Geometry check sheet. Reference: the model listing, model coordinates, mm. A direction names the side the tool comes from. Give positions to 0.01 mm unless a question says otherwise; leave off trailing zeros. Loops run counter-clockwise (first coordinate to the right, second up) from the corner with the lowest first, then second, coordinate; pieces in that order, holes last. Notation, with made-up numbers: (29, 85.5) - (76, 85.5) arc R20 cw to (76, 91.5) - close; hole circle Ø2 at (87.25, 71). An arc over 180 degrees is marked (long way). One line per question, with ' | ' between items. Start each with the question number.
Autodesk Inventor part; units mm, degrees
ref_plane "YZ Plane" through (0, 0, 0) normal (1, 0, 0) x (0, 1, 0)
ref_plane "XZ Plane" through (0, 0, 0) normal (0, 1, 0) x (-1, 0, 0)
ref_plane "XY Plane" through (0, 0, 0) normal (0, 0, 1) x (1, 0, 0)
sketch "Sketch1" plane through (0, 0, 0) normal (0, 0, 1) x (1, 0, 0)
  line L0 (0, 0) -> (50.8, 0)
  line L1 (50.8, 0) -> (50.8, 25.4)
  line L2 (50.8, 25.4) -> (0, 25.4)
  line L3 (0, 25.4) -> (0, 0)
  line L4 (1.905, 23.495) -> (48.895, 23.495)
  line L5 (48.895, 23.495) -> (48.895, 1.905)
  line L6 (48.895, 1.905) -> (1.905, 1.905)
  line L7 (1.905, 1.905) -> (1.905, 23.495)
  dimension "d0" = 50.8
  dimension "d1" = 25.4
  dimension "d2" = 1.905
extrude "Extrusion1" add sketch "Sketch1" along normal blind 330.2
sketch "Sketch2" plane through (0, 25.4, 0) normal (0, 1, 0) x (1, 0, 0)
  line L0 (1.905, -330.2) -> (48.895, -330.2) construction
  line L1 (25.4, -330.2) -> (25.4, -304.8) construction
  line L2 (25.4, -304.8) -> (25.4, -228.6) construction
  line L3 (50.8, 0) -> (0, 0) construction
  line L4 (25.4, 0) -> (25.4, -25.4) construction
  circle A0 centre (25.4, -304.8) radius 14.2748
  circle A1 centre (25.4, -25.4) radius 14.2875
  line L5 (25.4, -228.6) -> (12.7, -228.6) construction
  line L6 (12.7, -228.6) -> (25.4, -228.6) construction
  line L7 (25.4, -228.6) -> (38.1, -228.6) construction
  circle A2 centre (12.7, -228.6) radius 2.5797
  circle A3 centre (38.1, -228.6) radius 2.5797
  dimension "d5" = 25.4
  dimension "d6" = 76.2
  dimension "d7" = 25.4
  dimension "d8" = 28.5496
  dimension "d9" = 28.575
  dimension "d10" = 12.7
  dimension "d11" = 12.7
  dimension "d12" = 5.1594
  dimension "d13" = 5.1594
extrude "Extrusion2" cut sketch "Sketch2" against normal blind 355.6
properties part number "arm"
(1) Section check C-C, the plane z = 304.8. Record the boundary of the cut face in (x, y) (3 decimals), and give its area (3 significant figures).
(2) Section check B-B, the plane y = 6.25. Record the boundary of the cut face in (x, z) (3 decimals).
(3) Section check D-D, the plane z = 180. Record the boundary of the cut face in (x, y) (3 decimals).
(4) Depth check by flat-ended pin: pin 1 Ø17 at (x, z) = (25.4, 304.8) entering from -Y. Enter the tip coordinate at first touch or a pass-through.
(5) Section check A-A, the plane x = 25.4. Record the boundary of the cut face in (y, z) (1 decimal).
(6) Material ranges on line 1 (Z direction, x = 25.4, y = 0.5); line 2 (X direction, y = 1.25, z = 228.6); line 3 (X direction, y = 7.5, z = 53) (3 decimals), recorded low to high.
(7) Mould release check, pull along Y, two halves, no side actions. Record for faces 3 (the face through (0, 13, 163)), 4 (the face through (25, 23.495, 163)), 5 (the face through (25, 0, 163)): pulls with the +Y half, pulls with the -Y half, needs draft (parallel to the pull), parting line crosses it, or undercut.
(8) Tool access check on faces 1 (the face through (23.542, 24.461, 290.647)), 2 (the face through (26, 1.905, 163)). Record the directions out of +Z, -Z, +X, -X, +Y, -Y that give a thin tool (end or side, any length) a straight path to the whole face; none if there is none.
Numbers:
1) outline: (0, 0) - (11.125, 0) - (11.125, 1.905) - (1.905, 1.905) - (1.905, 23.495) - (11.125, 23.495) - (11.125, 25.4) - (0, 25.4) - close; (39.675, 0) - (50.8, 0) - (50.8, 25.4) - (39.675, 25.4) - (39.675, 23.495) - (48.895, 23.495) - (48.895, 1.905) - (39.675, 1.905) - close | area: 167 mm^2
2) outline: (0, 0) - (1.905, 0) - (1.905, 330.2) - (0, 330.2) - close; (48.895, 0) - (50.8, 0) - (50.8, 330.2) - (48.895, 330.2) - close
3) outline: (0, 0) - (50.8, 0) - (50.8, 25.4) - (0, 25.4) - close; hole (1.905, 1.905) - (48.895, 1.905) - (48.895, 23.495) - (1.905, 23.495) - close
4) pin 1: through
5) outline: (0, 0) - (1.9, 0) - (1.9, 11.1) - (0, 11.1) - close; (0, 39.7) - (1.9, 39.7) - (1.9, 290.5) - (0, 290.5) - close; (0, 319.1) - (1.9, 319.1) - (1.9, 330.2) - (0, 330.2) - close; (23.5, 0) - (25.4, 0) - (25.4, 11.1) - (23.5, 11.1) - close; (23.5, 39.7) - (25.4, 39.7) - (25.4, 290.5) - (23.5, 290.5) - close; (23.5, 319.1) - (25.4, 319.1) - (25.4, 330.2) - (23.5, 330.2) - close
6) line 1: 0 to 11.11, 39.69 to 290.53, 319.07 to 330.2 | line 2: 0 to 10.12, 15.28 to 35.52, 40.68 to 50.8 | line 3: 0 to 1.905, 48.895 to 50.8
7) face 3: needs draft | face 4: undercut | face 5: pulls with the -Y half
8) face 1: +Y, -Y | face 2: +Z, -Z
